```python
from build123d import *

# Parameters (mm, degrees)
BOSS_EXTRUDE1_DEPTH      = 15
BOSS_EXTRUDE1_DEPTH_BACK = 15
SKETCH2_R                = 1
CUT_EXTRUDE1_DEPTH       = 62.933569598
FILLET1_R                = 30
FILLET2_R                = 10


with BuildPart() as part:
    # Sketch1 → Boss-Extrude1 (new, two sides: drawn at the far end of the back side and taken through both)
    with BuildSketch(Plane(origin=(0, 0, 0), x_dir=(1, 0, 0), z_dir=(0, 1, 0)).offset(-BOSS_EXTRUDE1_DEPTH_BACK)):
        with BuildLine():
            Line((2.436698586, 0.75), (60.026698586, 0.75))
            Line((60.026698586, 0.75), (60.026698586, -0.75))
            Line((60.026698586, -0.75), (2.436698586, -0.75))
            ThreePointArc((2.436698586, -0.75), (1.980263122, -0.860243479), (1.624465724, -1.166666667))
            ThreePointArc((1.624465724, -1.166666667), (-2, 0), (1.624465724, 1.166666667))
            ThreePointArc((1.624465724, 1.166666667), (1.980263122, 0.860243479), (2.436698586, 0.75))
        make_face()
    extrude(amount=BOSS_EXTRUDE1_DEPTH + BOSS_EXTRUDE1_DEPTH_BACK)

    # Sketch2 → Cut-Extrude1 (cut, through all)
    with BuildSketch(Plane.XY.offset(0.75)):
        with Locations((49.952698586, 5)):
            Circle(SKETCH2_R)
        with Locations((45.952698586, 5)):
            Circle(SKETCH2_R)
        with Locations((41.952698586, 5)):
            Circle(SKETCH2_R)
        with Locations((37.952698586, 5)):
            Circle(SKETCH2_R)
        with Locations((33.952698586, 5)):
            Circle(SKETCH2_R)
        with Locations((29.952698586, 5)):
            Circle(SKETCH2_R)
        with Locations((25.952698586, 5)):
            Circle(SKETCH2_R)
        with Locations((21.952698586, 5)):
            Circle(SKETCH2_R)
        with Locations((45.952698586, -5)):
            Circle(SKETCH2_R)
        with Locations((41.952698586, -5)):
            Circle(SKETCH2_R)
        with Locations((37.952698586, -5)):
            Circle(SKETCH2_R)
        with Locations((33.952698586, -5)):
            Circle(SKETCH2_R)
        with Locations((29.952698586, -5)):
            Circle(SKETCH2_R)
        with Locations((25.952698586, -5)):
            Circle(SKETCH2_R)
        with Locations((21.952698586, -5)):
            Circle(SKETCH2_R)
        with Locations((49.952698586, -5)):
            Circle(SKETCH2_R)
        Polygon((49.952698586, 10), (21.952698586, 10), (2.940698586, 15), (60.026698586, 15), (60.026698586, 5), align=None)
        Polygon((49.952698586, -10), (21.952698586, -10), (2.940698586, -15), (60.026698586, -15), (60.026698586, -5), align=None)
    extrude(amount=-CUT_EXTRUDE1_DEPTH, mode=Mode.SUBTRACT)

    # Fillet1
    fillet1_edges = [part.edges().sort_by_distance(p)[0] for p in [
        (49.952698586, 10, 0),
        (21.952698586, 10, 0),
        (49.952698586, -10, 0),
        (21.952698586, -10, 0),
    ]]
    fillet(fillet1_edges, radius=FILLET1_R)

    # Fillet2
    # the kernel refuses this fillet: 10 mm, written as the material it takes off along each edge
    with BuildSketch(Plane(origin=(60.026698586, -5, 18.566207641), x_dir=(-0.9044112472912746, -0.4266618049146664, 0), z_dir=(0, 0, -1))) as fillet2_piece_1:
        with BuildLine():
            CenterArc((6.353468821, 9.970077682), FILLET2_R, 205.255895662, 69.177572528)
            Line((-2.690643652, 5.703459633), (-3.595054899, 5.276797828))
            Line((-3.595054899, 5.276797828), (-0.904411247, -0.426661805))
            Line((-0.904411247, -0.426661805), (-0.019905188, -0.999801872))
            ThreePointArc((-0.019905188, -0.999801872), (4.190379521, -1.083624989), (7.20378448, -0.997007768))
            Line((7.20378448, -0.997007768), (7.126483056, 0))
        make_face()
    extrude(amount=37.132415281, mode=Mode.SUBTRACT)
    with BuildSketch(Plane(origin=(60.026698586, 5, 18.566207641), x_dir=(0, -1, 0), z_dir=(0, 0, -1))) as fillet2_piece_2:
        with BuildLine():
            CenterArc((6.306267918, 10), FILLET2_R, 200.822427472, 69.177572528)
            Line((-3.040598123, 6.44527143), (-3.975284728, 6.089798573))
            ThreePointArc((-3.975284728, 6.089798573), (-2.767917517, 3.327484976), (-0.895739275, -0.444579747))
            Line((-0.895739275, -0.444579747), (0, -1))
            Line((0, -1), (6.306267918, -1))
            Line((6.306267918, -1), (6.306267918, 0))
        make_face()
    extrude(amount=37.132415281, mode=Mode.SUBTRACT)


solid = part.part
```
Verification items for the finished model (mm, model axes). A direction names the side the tool comes from. Coordinates: 2 decimals unless noted, no trailing zeros. Write each loop counter-clockwise with the first axis right and the second up, starting at its lowest first coordinate (ties: lowest second). Pieces come first, ordered by that corner, then holes. Notation, with made-up numbers: M 47,85 L 84,85 A25 ccw 84,120 Z; hole C -7,-29.75 d11. An arc over 180 degrees is marked long. Answer as a JSON object with one key per item and string values. Group by question number.
(1) Gauge pin test, flat ends, axial feed: pin 1 (0.8 mm diameter, centred on x = 33, z = 0, fed in from +Y); pin 2 (1.2 mm diameter, centred on x = 21.95, y = -5, fed in from -Z); pin 3 (2.5 mm diameter, centred on x = 41.95, y = -5, fed in from +Z); pin 4 (15 mm diameter, centred on x = 42.5, y = -6, fed in from -Z). Record the tip position at first contact, or that the pin passes through.
(2) Material ranges on line 1 (Z direction, x = 31.5, y = -3.75); line 2 (Y direction, x = 18.5, z = 0.05); line 3 (Y direction, x = 56.5, z = -0.3), recorded low to high.
(3) Release check for a two-part mould opening along Y. For faces 4 (the face through (41.22, -4.32, 0.01)), 5 (the face through (0, -15, 0)), 6 (the face through (48.414, 9.492, -0.01)) record: +Y half, -Y half, draft (parallel to the pull), parting line (faces both ways), or undercut.
(4) Cross-section at B-B, the plane x = 11.5. Record the cut outline in (y, z).
(5) Tool access check on faces 1 (the face through (24, 0, -0.75)), 2 (the face through (34, 10, 0)), 3 (the face through (48.26, -9.52, -0.01)). Record the directions out of +Z, -Z, +X, -X, +Y, -Y that give a thin tool (end or side, any length) a straight path to the whole face; none if there is none.
(6) Cross-section at C-C, the plane y = -5. State how many separate pieces and enclosed holes the cut face has, and give its area (3 significant figures).
(7) Cross-section at A-A, the plane y = 7. Record the cut outline in (x, z) (3 decimals), and give its area (3 significant figures).
(8) Cross-section at D-D, the plane y = -0.75. Record the cut outline in (x, z).
Reply:
{
 "1": {"pin 1": "y = 10", "pin 2": "through", "pin 3": "z = 0.75", "pin 4": "z = -0.75"},
 "2": {"line 1": "-0.75 to 0.75", "line 2": "-10.91 to 10.91", "line 3": "-6.32 to 6.32"},
 "3": {"face 4": "undercut", "face 5": "-Y half", "face 6": "+Y half"},
 "4": {"outline": "M -12.75,-0.75 L 12.75,-0.75 L 12.75,0.75 L -12.75,0.75 Z"},
 "5": {"face 1": "-Z, +X, +Y, -Y", "face 2": "+Z, -Z, +X, +Y", "face 3": "+Z, -Z, +X, -Y"},
 "6": {"separate pieces": "9", "enclosed holes": "0", "area": "72.4 mm²"},
 "7": {"outline": "M 1.624,-1.167 A1 cw 2.437,-0.75 L 55.595,-0.75 L 55.595,0.75 L 2.437,0.75 A1 cw 1.624,1.167 A2 ccw long Z", "area": "93.1 mm²"},
 "8": {"outline": "M 1.62,-1.17 A1 cw 2.44,-0.75 L 59.81,-0.75 L 59.81,0.75 L 2.44,0.75 A1 cw 1.62,1.17 A2 ccw long Z"}
}
